from build123d import *

# Parameters (mm, degrees)
F1_DEPTH = 5
F3_DEPTH = 6
F4_R     = 3
F5_DEPTH = 5
F6_R     = 4.7014922297
F7_DEPTH = 25


# Not quite as in the source:
# - a feature names something its author has since deleted; it is built from what else it names


with BuildPart() as f1:
    # F0 (on Front) → F1 (new body)
    with BuildSketch(Plane.XZ):
        with BuildLine():
            Line((-13.5, 0), (0, 0))
            Line((0, 0), (12.5000002478, 0))
            ThreePointArc((12.5000002478, 0), (16.0355341537, 1.4644660941), (17.5000002478, 5))
            Line((17.5000002478, 5), (17.5000002478, 15.5))
            ThreePointArc((17.5000002478, 15.5), (16.0355341537, 19.0355339059), (12.5000002478, 20.5))
            Line((12.5000002478, 20.5), (0, 20.5))
            Line((0, 20.5), (-13.5, 20.5))
            ThreePointArc((-13.5, 20.5), (-17.0355339059, 19.0355339059), (-18.5, 15.5))
            Line((-18.5, 15.5), (-18.5, 5))
            ThreePointArc((-18.5, 5), (-17.0355339059, 1.4644660941), (-13.5, 0))
        make_face()
    extrude(amount=F1_DEPTH)

    # F2 (on Right) → F3 (join, symmetric)
    with BuildSketch(Plane.YZ):
        with BuildLine():
            Line((0, 4.0980060585), (0, 0))
            Line((0, 0), (32, 0))
            ThreePointArc((32, 0), (32.4704336179, 2.5533766687), (31.6014834029, 5))
            Line((31.6014834029, 5), (22.881918614, 5))
            Line((22.881918614, 5), (0, 5))
            Line((0, 5), (0, 4.0980060585))
        make_face()
        with BuildLine():
            Line((32, 20.5), (0, 20.5))
            Line((0, 20.5), (0, 15.5))
            Line((0, 15.5), (32, 15.5))
            ThreePointArc((32, 15.5), (33.3190218942, 18), (32, 20.5))
        make_face()
    extrude(amount=F3_DEPTH, both=True)

    # F4 (on face) → F5 (cut)
    with BuildSketch(Plane(origin=(0, 0, 0), x_dir=(-1, 0, 0), z_dir=(0, 1, 0))):
        with Locations((12.4534495048, 16.4442711417)):
            Circle(F4_R)
        with Locations((12.4534495048, 3.7959093649)):
            Circle(F4_R)
        with Locations((-12.5748278123, 16.4442711417)):
            Circle(F4_R)
        with Locations((-12.5748278123, 3.7959093649)):
            Circle(F4_R)
    extrude(amount=-F5_DEPTH, mode=Mode.SUBTRACT)

    # F6 (on face) → F7 (cut)
    with BuildSketch(Plane.XY.offset(20.5)):
        with Locations((0, 26.9046556205)):
            Circle(F6_R)
    extrude(amount=-F7_DEPTH, mode=Mode.SUBTRACT)


solid = f1.part
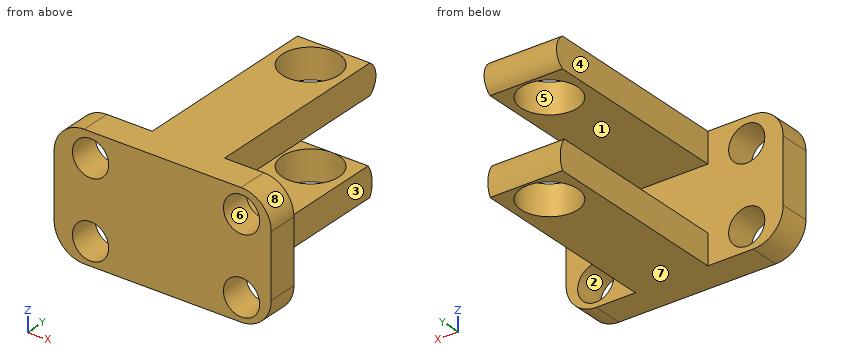
Geometry check sheet. Reference: the model listing, model coordinates, mm. Face numbers are marked on the shaded views. A direction names the side the tool comes from. Give positions to 0.01 mm unless a question says otherwise; leave off trailing zeros. Order: outer loops, then holes, each group sorted by start corner. A loop starts at its lowest first (then second) coordinate and runs counter-clockwise, first axis right, second up.
1) Material ranges on probe 1 along Y at (x, z) = (0, 18.15); probe 2 along Z at (x, y) = (-2, 9.5); probe 3 along X at (y, z) = (21, 16.25), recorded low to high.
Results are:
probe 1: y = -5 to 22.2, 31.61 to 33.32
probe 2: z = 0 to 5, 15.5 to 20.5
probe 3: x = -6 to 6
2) Draft check along X on the marked faces 6, 7 and 8. Enter one of: released by +X, released by -X, zero draft, split by the parting line, or undercut.
Results are:
face 6: undercut
face 7: zero draft
face 8: released by +X
3) Gauge pin test, flat ends, axial feed: pin 1 (5.5 mm diameter, centred on y = 20, z = 1.5, fed in from +X); pin 2 (2 mm diameter, centred on x = -13.5, z = 7.5, fed in from +Y); pin 3 (1.5 mm diameter, centred on y = 11, z = 3, fed in from -X); pin 4 (4 mm diameter, centred on y = 0.5, z = 9.5, fed in from -X). Record the tip position at first contact, or that the pin passes through.
Results are:
pin 1: stops at x = 6
pin 2: stops at y = 0
pin 3: stops at x = -6
pin 4: stops at x = -18.5
4) Cross-section at A-A (y = 14). Record the boundary of the cut face in (x, z), then the cut area to 3 significant figures.
Results are:
outline: (-6, 0) - (6, 0) - (6, 5) - (-6, 5) - close; (-6, 15.5) - (6, 15.5) - (6, 20.5) - (-6, 20.5) - close
area: 120 mm2
5) Cross-section at D-D (y = 23). Record the boundary of the cut face in (x, z), then the cut area to 3 significant figures.
Results are:
outline: (-6, 0) - (-2.62, 0) - (-2.62, 5) - (-6, 5) - close; (-6, 15.5) - (-2.62, 15.5) - (-2.62, 20.5) - (-6, 20.5) - close; (2.62, 0) - (6, 0) - (6, 5) - (2.62, 5) - close; (2.62, 15.5) - (6, 15.5) - (6, 20.5) - (2.62, 20.5) - close
area: 67.6 mm2
6) Cross-section at C-C (x = 13.5). Record the boundary of the cut face in (y, z).
Results are:
outline: (-5, 0.1) - (0, 0.1) - (0, 0.94) - (-5, 0.94) - close; (-5, 6.65) - (0, 6.65) - (0, 13.59) - (-5, 13.59) - close; (-5, 19.3) - (0, 19.3) - (0, 20.4) - (-5, 20.4) - close
7) Cross-section at B-B (z = 14.25). Record the boundary of the cut face in (x, y).
Results are:
outline: (-18.5, -5) - (-14.5, -5) - (-14.5, 0) - (-18.5, 0) - close; (-10.41, -5) - (10.53, -5) - (10.53, 0) - (-10.41, 0) - close; (14.62, -5) - (17.5, -5) - (17.5, 0) - (14.62, 0) - close
8) Tool access check on the marked faces 1, 2, 3, 4 and 5. Record the directions out of +Z, -Z, +X, -X, +Y, -Y that give a thin tool (end or side, any length) a straight path to the whole face; none if there is none.
Results are:
face 1: +X, -X, +Y
face 2: +Y, -Y
face 3: +Z, -Z, +X, +Y
face 4: +Z, -Z, -X, +Y
face 5: +Z, -Z
